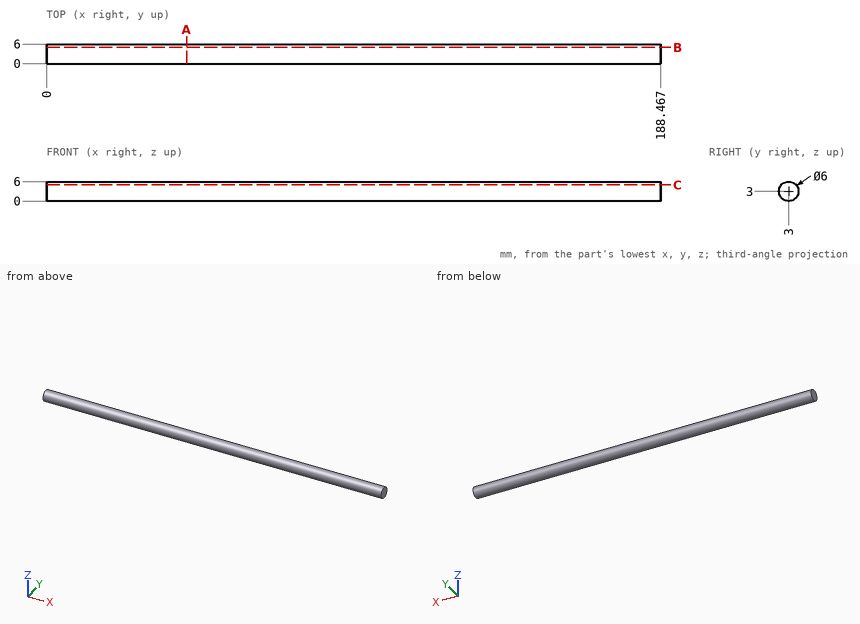
Study the drawing (mm; zero at the part's minimum x, y, z) and answer. Coordinates: 2 decimals unless noted, no trailing zeros. Loops run counter-clockwise (first coordinate to the right, second up) from the corner with the lowest first, then second, coordinate; pieces in that order, holes last. Notation, with made-up numbers: (36.25, 38) -> (72.25, 38) arc R22 cw to (72.25, 57) -> close; hole circle Ø3 at (87.25, 60). An arc over 180 degrees is marked (long way). Write each question's results on one line, items separated by ' | '. Start each with the question number.
1) A flat-ended cylindrical pin translates along its axis: P1, Ø1.5, axis at x = 36.5, y = 2, coming from the +Z side. Find the tip coordinate at first contact, or state that the pin passes through.
2) Find section B-B on y = 5. Determine the outline of the cut face in (x, z).
3) Consider line 1 along Y through (x, z) = (171, 2.7) (1 decimal); line 2 along Y through (x, z) = (112, 1.3). Determine where each line is inside the solid, lowest interval first.
4) Find section A-A on x = 43. Determine the outline of the cut face in (y, z), then the cut area to 3 significant figures.
Response values:
1) P1: stops at z = 5.99
2) outline: (0, 0.76) -> (188.47, 0.76) -> (188.47, 5.24) -> (0, 5.24) -> close
3) line 1: y = 0 to 6 | line 2: y = 0.53 to 5.47
4) outline: circle Ø6 at (3, 3) | area: 28.3 mm^2
